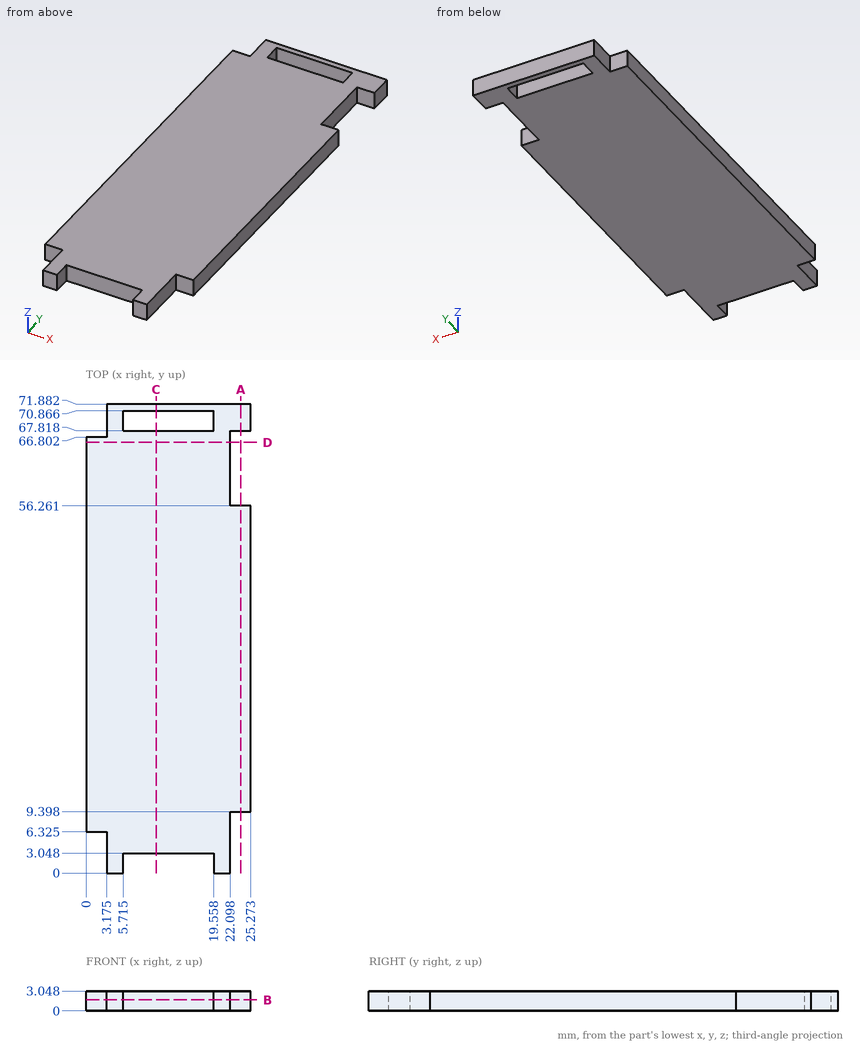
The figure shows three views and two pictorial views of one solid part (mm, origin at its lowest corner). Answer the questions. Coordinates: 2 decimals unless noted, no trailing zeros. Write each loop counter-clockwise with the first axis right and the second up, starting at its lowest first coordinate (ties: lowest second). Pieces come first, ordered by that corner, then holes. Notation, with made-up numbers: (63.5, -34) -> (96.5, -34) arc R27 cw to (96.5, -1) -> close; hole circle Ø8 at (87, -3.5). An arc over 180 degrees is marked (long way). Return JSON: item names as keys, results as strings.
1. A cutting plane is placed at D-D (y = 66). Determine the outline of the cut face in (x, z).
Found:
{"outline": "(0, 0) -> (22.1, 0) -> (22.1, 3.05) -> (0, 3.05) -> close"}
2. Each of these flat-tipped pins is pushed along its axis until it touches: P1, Ø1, axis at x = 6.5, z = 1, coming from the -Y side; P2, Ø0.9, axis at y = 1.5, z = 1, coming from the -X side (3 decimals); P3, Ø1.5, axis at y = 3, z = 2, coming from the +X side. Where does it stop, or does it pass through?
Found:
{"P1": "y = 3.05", "P2": "x = 3.175", "P3": "x = 22.1"}
3. Find the intervals of material crossed by line 1 along Y through (x, z) = (12.75, 1.05); line 2 along X through (y, z) = (5, 1.7) (1 decimal); line 3 along X through (y, z) = (58, 0.15), in increasing order. Write a range as from..to.
Found:
{"line 1": "3.05..67.82, 70.87..71.88", "line 2": "3.2..22.1", "line 3": "0..22.1"}
4. A cutting plane is placed at B-B (z = 1.7). Determine the outline of the cut face in (x, y) (1 decimal), and give its area (3 significant figures).
Found:
{"outline": "(0, 6.3) -> (3.2, 6.3) -> (3.2, 0) -> (5.7, 0) -> (5.7, 3) -> (19.6, 3) -> (19.6, 0) -> (22.1, 0) -> (22.1, 9.4) -> (25.3, 9.4) -> (25.3, 56.3) -> (22.1, 56.3) -> (22.1, 67.8) -> (25.3, 67.8) -> (25.3, 71.9) -> (3.2, 71.9) -> (3.2, 66.8) -> (0, 66.8) -> close; hole (5.7, 67.8) -> (19.6, 67.8) -> (19.6, 70.9) -> (5.7, 70.9) -> close", "area": "1,630 mm2"}
5. A cutting plane is placed at C-C (x = 10.75). Determine the outline of the cut face in (y, z).
Found:
{"outline": "(3.05, 0) -> (67.82, 0) -> (67.82, 3.05) -> (3.05, 3.05) -> close; (70.87, 0) -> (71.88, 0) -> (71.88, 3.05) -> (70.87, 3.05) -> close"}
6. A cutting plane is placed at A-A (x = 23.75). Determine the outline of the cut face in (y, z), and give its area (3 significant figures).
Found:
{"outline": "(9.4, 0) -> (56.26, 0) -> (56.26, 3.05) -> (9.4, 3.05) -> close; (67.82, 0) -> (71.88, 0) -> (71.88, 3.05) -> (67.82, 3.05) -> close", "area": "155 mm2"}
